Input: part model. Units: mm. Frame: model coordinates. A direction names the side the tool comes from. Give positions to 0.01 mm unless a question says otherwise; leave off trailing zeros. Loops run counter-clockwise (first coordinate to the right, second up) from the corner with the lowest first, then second, coordinate; pieces in that order, holes last. Notation, with made-up numbers: (57, -2.5) - (113, -2.5) arc R24 ccw to (113, 8.5) - close; hole circle Ø10 at (43, 36). An arc over 180 degrees is marked (long way). One line per item, written item: value.
from build123d import *

# Parameters (mm, degrees)
SKETCH_1_W          = 40
SKETCH_1_H          = 20
SKETCH_1_W_2        = 38
SKETCH_1_H_2        = 18
EXTRUDE_1_DEPTH     = 115
SKETCH_2_R          = 2
CUT_EXTRUDE_1_DEPTH = 115
SKETCH_3_R          = 2.025
CUT_EXTRUDE_2_DEPTH = 35
CUT_EXTRUDE_3_DEPTH = 129.5
CUT_EXTRUDE_4_DEPTH = 129.5


with BuildPart() as part:
    # 草图1 → 凸台-拉伸1 (new, symmetric)
    with BuildSketch(Plane.XY):
        Rectangle(SKETCH_1_W, SKETCH_1_H)
        Rectangle(SKETCH_1_W_2, SKETCH_1_H_2, mode=Mode.SUBTRACT)
    extrude(amount=EXTRUDE_1_DEPTH, both=True)

    # 草图2 → 切除-拉伸1 (cut, symmetric)
    with BuildSketch(Plane(origin=(0, 10, 0), x_dir=(1, 0, 0), z_dir=(0, 1, 0))):
        with Locations((-15, 105)):
            Circle(SKETCH_2_R)
        with Locations((15, 105)):
            Circle(SKETCH_2_R)
    cut_extrude_1 = extrude(amount=CUT_EXTRUDE_1_DEPTH, both=True, mode=Mode.SUBTRACT)

    # 镜向1: 切除-拉伸1 across plane
    add(cut_extrude_1.mirror(Plane.XY), mode=Mode.SUBTRACT)

    # 草图3 → 切除-拉伸2 (cut, symmetric)
    with BuildSketch(Plane.XZ.offset(10)):
        with Locations(Location((-13.975679885, -47.500000831, 0), (0, 0, 270))):
            Circle(SKETCH_3_R)
        with Locations(Location((11.024320115, -47.500000831, 0), (0, 0, 270))):
            Circle(SKETCH_3_R)
        with Locations(Location((-13.975679885, 47.499999169, 0), (0, 0, 270))):
            Circle(SKETCH_3_R)
        with Locations(Location((11.024320115, 47.499999169, 0), (0, 0, 270))):
            Circle(SKETCH_3_R)
    extrude(amount=CUT_EXTRUDE_2_DEPTH, both=True, mode=Mode.SUBTRACT)

    # 草图4 → 切除-拉伸3 (cut, symmetric)
    with BuildSketch(Plane(origin=(20, 0, 0), x_dir=(0, 0, -1), z_dir=(1, 0, 0))):
        with BuildLine():
            Line((-30, 5), (30, 5))
            ThreePointArc((30, 5), (35, 0), (30, -5))
            Line((30, -5), (-30, -5))
            ThreePointArc((-30, -5), (-35, 0), (-30, 5))
        make_face()
    extrude(amount=CUT_EXTRUDE_3_DEPTH, both=True, mode=Mode.SUBTRACT)

    # 草图5 → 切除-拉伸4 (cut, symmetric)
    with BuildSketch(Plane(origin=(20, 0, 0), x_dir=(0, 0, -1), z_dir=(1, 0, 0))):
        with BuildLine():
            Line((-86.249999585, 5), (-66.249999585, 5))
            ThreePointArc((-66.249999585, 5), (-61.249999585, 0), (-66.249999585, -5))
            Line((-66.249999585, -5), (-86.249999585, -5))
            ThreePointArc((-86.249999585, -5), (-91.249999585, 0), (-86.249999585, 5))
        make_face()
    cut_extrude_4 = extrude(amount=CUT_EXTRUDE_4_DEPTH, both=True, mode=Mode.SUBTRACT)

    # 镜向2: 切除-拉伸4 across plane
    add(cut_extrude_4.mirror(Plane.XY), mode=Mode.SUBTRACT)


solid = part.part
Item 1: Section A-A, the plane z = 19. Output: boundary loops of the cut face in (x, y), and give its area (3 significant figures).
Verdict:
outline: (-20, -10) - (20, -10) - (20, -5) - (19, -5) - (19, -9) - (-19, -9) - (-19, -5) - (-20, -5) - close; (-20, 5) - (-19, 5) - (-19, 9) - (19, 9) - (19, 5) - (20, 5) - (20, 10) - (-20, 10) - close
area: 96.0 mm^2
Item 2: Material intervals for L1, parallel to X at y = -9.35, z = -105; L2, parallel to X at y = -9.25, z = -47.5; L3, parallel to Y at x = 7.5, z = 5.5, sorted ascending.
Verdict:
L1: x = -20 to -17, -13 to 13, 17 to 20
L2: x = -20 to -16, -11.95 to 9, 13.05 to 20
L3: y = -10 to -9, 9 to 10
Item 3: Access query for faces 3 (the face through (19.5, 0.1, -35)), 4 (the face through (0, 9, 2)), 5 (the face through (9.792, -9.507, -45.893)). Directions: +Z, -Z, +X, -X, +Y, -Y. A direction counts if a zero-diameter tool reaches every point of the face in a straight line with its end or side. Return the directions, or none.
Verdict:
face 3: +X, -X
face 4: +Z, -Z
face 5: +Y, -Y
Item 4: Section D-D, the plane x = 2.5. Output: boundary loops of the cut face in (y, z), and give its area (3 significant figures).
Verdict:
outline: (-10, -115) - (-9, -115) - (-9, 115) - (-10, 115) - close; (9, -115) - (10, -115) - (10, 115) - (9, 115) - close
area: 460 mm^2
Item 5: Draft query along Z for faces 1 (the face through (-12.607, 9.493, 48.993)), 2 (the face through (-19, -6, 2)). Return one class per face: pulls with the +Z half, pulls with the -Z half, needs draft (parallel to the pull), parting line crosses it, or undercut.
Verdict:
face 1: undercut
face 2: needs draft
Item 6: Section C-C, the plane z = 105. Output: boundary loops of the cut face in (x, y).
Verdict:
outline: (-20, -10) - (-17, -10) - (-17, -9) - (-19, -9) - (-19, 9) - (-17, 9) - (-17, 10) - (-20, 10) - close; (-13, -10) - (13, -10) - (13, -9) - (-13, -9) - close; (-13, 9) - (13, 9) - (13, 10) - (-13, 10) - close; (17, -10) - (20, -10) - (20, 10) - (17, 10) - (17, 9) - (19, 9) - (19, -9) - (17, -9) - close
Item 7: Section B-B, the plane y = 0. Count the separate pieces of the cut face and the enclosed holes in it, and give its area (3 significant figures).
Verdict:
separate pieces: 8
enclosed holes: 0
area: 200 mm^2
